from build123d import *

# Parameters (mm, degrees)
SKETCH1_W                                     = 50.386
SKETCH1_H                                     = 90.518
SKETCH1_W_2                                   = 40.386
SKETCH1_H_2                                   = 80.518
BOSS_EXTRUDE1_DEPTH                           = 101.6
SKETCH2_W                                     = 101.186
SKETCH2_H                                     = 141.318
BOSS_EXTRUDE2_DEPTH                           = 10
FILLET1_R                                     = 12
CBORE_FOR_6_BINDING_HEAD_MACHINE_SC_2_R       = 1.89865
CBORE_FOR_6_BINDING_HEAD_MACHINE_SCREW2_DEPTH = 10
CBORE_START                                   = 7.7902
CBORE_FOR_6_BINDING_HEAD_MACHINE_SC_3_O_R     = 3.96875
CBORE_FOR_6_BINDING_HEAD_MACHINE_SC_3_O_R_2   = 1.89865
CBORE_FOR_6_BINDING_HEAD_MACHINE_SC_3_DEPTH   = 2.2098
FILLET2_R                                     = 12
SKETCH9_R                                     = 3
CUT_EXTRUDE1_DEPTH                            = 163.231915396
CUT_EXTRUDE2_REACH                            = 135.697
SKETCH10_W                                    = 41.656
SKETCH10_H                                    = 81.788
SKETCH10_W_2                                  = 40.386
SKETCH10_H_2                                  = 80.518
CUT_EXTRUDE2_DIRECTION_2_DEPTH                = 134.697067769


# Read off the part's stored shape, not the designer's step: CBORE for #6 Binding Head Machine Screw2
with BuildPart() as part:
    # Sketch1 → Boss-Extrude1 (new body)
    with BuildSketch(Plane(origin=(0, 0, 0), x_dir=(1, 0, 0), z_dir=(0, 1, 0))):
        Rectangle(SKETCH1_W, SKETCH1_H)
        Rectangle(SKETCH1_W_2, SKETCH1_H_2, mode=Mode.SUBTRACT)
    extrude(amount=BOSS_EXTRUDE1_DEPTH)

    # Sketch2 → Boss-Extrude2 (add)
    with BuildSketch(Plane(origin=(0, 0, 0), x_dir=(1, 0, 0), z_dir=(0, 1, 0))):
        Rectangle(SKETCH2_W, SKETCH2_H)
    extrude(amount=BOSS_EXTRUDE2_DEPTH)

    # Fillet1
    fillet1_edges = [part.edges().sort_by_distance(p)[0] for p in [
        (0, 10, -45.259),
        (25.193, 10, 0),
        (0, 10, 45.259),
        (-25.193, 10, 0),
    ]]
    fillet(fillet1_edges, radius=FILLET1_R)

    # CBORE for _6 Binding Head Machine Sc 2 → CBORE for #6 Binding Head Machine Screw2 (cut)
    with BuildSketch(Plane(origin=(0, 0, 0), x_dir=(1, 0, 0), z_dir=(0, 1, 0))):
        with Locations((41.060456563, -60.576250035)):
            Circle(CBORE_FOR_6_BINDING_HEAD_MACHINE_SC_2_R)
        with Locations((-41.060456563, 60.576250035)):
            Circle(CBORE_FOR_6_BINDING_HEAD_MACHINE_SC_2_R)
        with Locations((-41.060456563, -60.576250035)):
            Circle(CBORE_FOR_6_BINDING_HEAD_MACHINE_SC_2_R)
        with Locations((41.060456563, 60.576250035)):
            Circle(CBORE_FOR_6_BINDING_HEAD_MACHINE_SC_2_R)
        Circle(CBORE_FOR_6_BINDING_HEAD_MACHINE_SC_2_R)
    extrude(amount=CBORE_FOR_6_BINDING_HEAD_MACHINE_SCREW2_DEPTH, mode=Mode.SUBTRACT)

    # CBORE for _6 Binding Head Machine Sc 3 o → CBORE for _6 Binding Head Machine Sc 3 (cut)
    # profile 1 of 5: a face of its own
    with BuildSketch(Plane(origin=(0, 0, 0), x_dir=(1, 0, 0), z_dir=(0, 1, 0)).offset(CBORE_START)):
        with Locations((41.060456563, -60.576250035)):
            Circle(CBORE_FOR_6_BINDING_HEAD_MACHINE_SC_3_O_R)
        with Locations((41.060456563, -60.576250035)):
            Circle(CBORE_FOR_6_BINDING_HEAD_MACHINE_SC_3_O_R_2, mode=Mode.SUBTRACT)
    # profile 2 of 5: a face of its own
    with BuildSketch(Plane(origin=(0, 0, 0), x_dir=(1, 0, 0), z_dir=(0, 1, 0)).offset(CBORE_START)):
        with Locations((-41.060456563, 60.576250035)):
            Circle(CBORE_FOR_6_BINDING_HEAD_MACHINE_SC_3_O_R)
        with Locations((-41.060456563, 60.576250035)):
            Circle(CBORE_FOR_6_BINDING_HEAD_MACHINE_SC_3_O_R_2, mode=Mode.SUBTRACT)
    # profile 3 of 5: a face of its own
    with BuildSketch(Plane(origin=(0, 0, 0), x_dir=(1, 0, 0), z_dir=(0, 1, 0)).offset(CBORE_START)):
        with Locations((-41.060456563, -60.576250035)):
            Circle(CBORE_FOR_6_BINDING_HEAD_MACHINE_SC_3_O_R)
        with Locations((-41.060456563, -60.576250035)):
            Circle(CBORE_FOR_6_BINDING_HEAD_MACHINE_SC_3_O_R_2, mode=Mode.SUBTRACT)
    # profile 4 of 5: a face of its own
    with BuildSketch(Plane(origin=(0, 0, 0), x_dir=(1, 0, 0), z_dir=(0, 1, 0)).offset(CBORE_START)):
        with Locations((41.060456563, 60.576250035)):
            Circle(CBORE_FOR_6_BINDING_HEAD_MACHINE_SC_3_O_R)
        with Locations((41.060456563, 60.576250035)):
            Circle(CBORE_FOR_6_BINDING_HEAD_MACHINE_SC_3_O_R_2, mode=Mode.SUBTRACT)
    # profile 5 of 5: a face of its own
    with BuildSketch(Plane(origin=(0, 0, 0), x_dir=(1, 0, 0), z_dir=(0, 1, 0)).offset(CBORE_START)):
        Circle(CBORE_FOR_6_BINDING_HEAD_MACHINE_SC_3_O_R)
        Circle(CBORE_FOR_6_BINDING_HEAD_MACHINE_SC_3_O_R_2, mode=Mode.SUBTRACT)
    extrude(amount=CBORE_FOR_6_BINDING_HEAD_MACHINE_SC_3_DEPTH, mode=Mode.SUBTRACT)

    # Fillet2
    fillet2_edges = [part.edges().sort_by_distance(p)[0] for p in [
        (50.593, 5, 70.659),
        (50.593, 5, -70.659),
        (-50.593, 5, -70.659),
        (-50.593, 5, 70.659),
    ]]
    fillet(fillet2_edges, radius=FILLET2_R)

    # Sketch9 → Cut-Extrude1 (cut, through all)
    with BuildSketch(Plane.XY.offset(45.259)):
        with Locations((0, 88.608727906)):
            Circle(SKETCH9_R)
        with Locations((0, 37.808727906)):
            Circle(SKETCH9_R)
    extrude(amount=-CUT_EXTRUDE1_DEPTH, mode=Mode.SUBTRACT)

    # Cut-Extrude2: up to this face of the body (flat: up to its plane)
    cut_extrude2_end = Plane(part.part.faces().sort_by_distance((0, 10, -39.358212715))[0])
    # Sketch10 → Cut-Extrude2 (cut, up to the picked face)
    with BuildSketch(Plane(origin=(0, 101.6, 0), x_dir=(1, 0, 0), z_dir=(0, 1, 0)), mode=Mode.PRIVATE) as cut_extrude2_sk1:
        Rectangle(SKETCH10_W, SKETCH10_H)
        Rectangle(SKETCH10_W_2, SKETCH10_H_2, mode=Mode.SUBTRACT)
    cut_extrude2_tool1 = split(extrude(cut_extrude2_sk1.sketch, amount=-CUT_EXTRUDE2_REACH, mode=Mode.PRIVATE), bisect_by=cut_extrude2_end, keep=Keep.BOTH, mode=Mode.PRIVATE)
    add(cut_extrude2_tool1.solids().sort_by(Axis((20.736215, 101.6, 0), (0, -1, 0)))[0], mode=Mode.SUBTRACT)

    # Sketch10 → Cut-Extrude2 direction 2 (cut)
    with BuildSketch(Plane(origin=(0, 101.6, 0), x_dir=(1, 0, 0), z_dir=(0, 1, 0))):
        Rectangle(SKETCH10_W, SKETCH10_H)
        Rectangle(SKETCH10_W_2, SKETCH10_H_2, mode=Mode.SUBTRACT)
    extrude(amount=CUT_EXTRUDE2_DIRECTION_2_DEPTH, mode=Mode.SUBTRACT)


solid = part.part
Part model, mm, in its own coordinate system. A direction names the side the tool comes from. Coordinates: 2 decimals unless noted, no trailing zeros. Order: outer loops, then holes, each group sorted by start corner. A loop starts at its lowest first (then second) coordinate and runs counter-clockwise, first axis right, second up. Notation, with made-up numbers: M 87.25,60 L 134.25,60 A23 cw 134.25,73 Z; hole C -35,29.5 d5. An arc over 180 degrees is marked long. One line per question, with ' | ' between items.
Q1. Two-plate mould, pull along Y, no slides. Class faces 1 (the face through (-0.65, 85.68, 43.11)), 2 (the face through (0, 61, -45.259)), 3 (the face through (-46, 10, -1)): +Y half, -Y half, draft (parallel to the pull), parting line (faces both ways), or undercut.
A:
face 1: undercut | face 2: draft | face 3: +Y half
Q2. Slice it at C-C (y = 50). Give the cut face in (x, z), and give its area (3 significant figures).
A:
outline: M -25.19,-45.26 L 25.19,-45.26 L 25.19,45.26 L -25.19,45.26 Z; hole M -20.83,-40.89 L 20.83,-40.89 L 20.83,40.89 L -20.83,40.89 Z | area: 1,150 mm^2
Q3. Slice it at B-B (x = -18). Give the cut face in (y, z).
A:
outline: M 0,-70.66 L 10,-70.66 L 10,-57.26 A12 cw 22,-45.26 L 101.6,-45.26 L 101.6,-40.89 L 10,-40.89 L 10,40.89 L 101.6,40.89 L 101.6,45.26 L 22,45.26 A12 cw 10,57.26 L 10,70.66 L 0,70.66 Z
Q4. Slice it at D-D (x = 0). Count the separate pieces of the cut face and the enclosed holes in it, and give its area (3 significant figures).
A:
separate pieces: 6 | enclosed holes: 0 | area: 2,120 mm^2
Q5. 3-axis set-ups, long thin cutter, end or side, ignore diameter. For faces 4 (the face through (1.8, 3.8, -0.6)), 5 (the face through (-38.927, 8.88, -63.923)), 6 (the face through (0, 61, 45.259)): which of +Z, -Z, +X, -X, +Y, -Y reach the whole face in a straight line?
A:
face 4: +Y, -Y | face 5: +Y | face 6: +Z, +X, -X, +Y
Q6. Drill centre lines: line 1 (X direction, y = 36, z = -19); line 2 (X direction, y = 6, z = 0); line 3 (Z direction, x = -22.5, y = 70). Where is each one in solid material? Low to high.
A:
line 1: x = -25.19 to -20.83, 20.83 to 25.19 | line 2: x = -50.59 to -1.9, 1.9 to 50.59 | line 3: z = -45.26 to 45.26
Q7. Slice it at A-A (z = 0). Give the cut face in (x, y).
A:
outline: M -50.59,0 L -1.9,0 L -1.9,7.79 L -3.97,7.79 L -3.97,10 L -20.83,10 L -20.83,101.6 L -25.19,101.6 L -25.19,22 A12 cw -37.19,10 L -50.59,10 Z; M 1.9,0 L 50.59,0 L 50.59,10 L 37.19,10 A12 cw 25.19,22 L 25.19,101.6 L 20.83,101.6 L 20.83,10 L 3.97,10 L 3.97,7.79 L 1.9,7.79 Z
Q8. Pin check, flat tips, straight feed: P1, Ø5, axis at x = 0, y = 37.81, coming from the +Z side; P2, Ø3, axis at x = -14.5, y = 71, coming from the -Z side; P3, Ø6.5, axis at x = 41, z = -62, coming from the +Y side; P4, Ø10, axis at y = 17, z = -24, coming from the +X side. Stop position of each tip, or through.
A:
P1: passes through | P2: stops at z = -45.26 | P3: stops at y = 10 | P4: stops at x = 30.56
